```python
from build123d import *

# Parameters (mm, degrees)
F0_W     = 87.63
F0_H     = 71.12
F1_DEPTH = 25.4
F2_W     = 74.929997
F2_H     = 58.42
F3_DEPTH = 24.13
F4_W     = 16.083958
F4_H     = 6.761409
F5_DEPTH = 7.62
F6_W     = 87.63
F6_H     = 1.905
F7_DEPTH = 5.08
F9_DEPTH = 5.08


with BuildPart() as f1:
    # F0 (on Top) → F1 (new body)
    with BuildSketch(Plane.XY):
        with Locations((-1.058847, -6.879137)):
            Rectangle(F0_W, F0_H)
    extrude(amount=F1_DEPTH)

    # F2 (on face) → F3 (cut)
    with BuildSketch(Plane.XY.offset(25.4)):
        with Locations((-1.058847, -6.879137)):
            Rectangle(F2_W, F2_H)
    extrude(amount=-F3_DEPTH, mode=Mode.SUBTRACT)

    # F4 (on face) → F5 (cut)
    with BuildSketch(Plane.YZ.offset(42.756153)):
        with Locations((8.041979, 15.468483)):
            Rectangle(F4_W, F4_H)
    extrude(amount=-F5_DEPTH, mode=Mode.SUBTRACT)

    # F6 (on face) → F7 (cut)
    with BuildSketch(Plane.XY.offset(25.4)):
        with Locations((-1.058847, 25.061363)):
            Rectangle(F6_W, F6_H)
        with Locations((-1.058847, -38.819637)):
            Rectangle(F6_W, F6_H)
    extrude(amount=-F7_DEPTH, mode=Mode.SUBTRACT)

    # F8 (on face) → F9 (join)
    with BuildSketch(Plane.XY.offset(12.087778)):
        Polygon((12.600807, 0), (36.406152, 0), (36.406152, 16.083958), (36.406152, 22.332337), (12.600807, 22.332337), align=None)
    extrude(amount=-F9_DEPTH)


solid = f1.part
```
The listing builds one solid part. Answer for the finished solid, in the listing's coordinates (mm). A direction names the side the tool comes from. Round coordinates to 2 decimals unless told otherwise and drop trailing zeros. Loops run counter-clockwise (first coordinate to the right, second up) from the corner with the lowest first, then second, coordinate; pieces in that order, holes last.
Q1. Section D-D, the plane x = 27 is taken. Determine the outline of the cut face in (y, z).
Q2. Given pin 1 Ø5 at (x, y) = (16, -23) entering from +Z; pin 2 Ø6.5 at (x, y) = (19, 8) entering from +Z, each flat-ended and moving along its own axis, determine where each tip first touches the part or whether it passes through.
Q3. Find the intervals of material crossed by line 1 (Y direction, x = 18.5, z = 20.75); line 2 (X direction, y = -2.5, z = 22.25); line 3 (Z direction, x = 21, y = 12.5), in increasing order.
Q4. Section A-A, the plane z = 21.25 is taken. Determine the outline of the cut face in (x, y), then the cut area to 3 significant figures.
Q5. For a pull along X with two mould halves and no side action, classify faces 6 (the face through (-44.874, -7, 13)), 7 (the face through (-2, -6, 0)), 8 (the face through (24, 11, 12.088)) as released by +X, released by -X, zero draft, split by the parting line, or undercut.
Q6. Which of the six approach directions +Z, -Z, +X, -X, +Y, -Y give full straight-line access (tool end or side, diameter ignored) to faces 1 (the face through (-2, -39.772, 23)), 2 (the face through (12.601, 11, 10)), 3 (the face through (40, 0, 15)), 4 (the face through (-1, 23, 25.4)), 5 (the face through (-2, -6, 1.27))?
Q7. Section B-B, the plane y = 11 is taken. Determine the outline of the cut face in (x, z), then the cut area to 3 significant figures.
Q8. Section C-C, the plane z = 10.75 is taken. Determine the outline of the cut face in (x, y), then the cut area to 3 significant figures.
Completed:
1. outline: (-42.44, 0) - (28.68, 0) - (28.68, 25.4) - (26.01, 25.4) - (26.01, 20.32) - (24.11, 20.32) - (24.11, 25.4) - (22.33, 25.4) - (22.33, 12.09) - (0, 12.09) - (0, 7.01) - (22.33, 7.01) - (22.33, 1.27) - (-36.09, 1.27) - (-36.09, 25.4) - (-37.87, 25.4) - (-37.87, 20.32) - (-39.77, 20.32) - (-39.77, 25.4) - (-42.44, 25.4) - close
2. pin 1: stops at z = 1.27
2. pin 2: stops at z = 12.09
3. line 1: y = -42.44 to -39.77, -37.87 to -36.09, 22.33 to 24.11, 26.01 to 28.68
3. line 2: x = -44.87 to -38.52, 36.41 to 42.76
3. line 3: z = 0 to 1.27, 7.01 to 12.09
4. outline: (-44.87, -42.44) - (42.76, -42.44) - (42.76, -39.77) - (-44.87, -39.77) - close; (-44.87, -37.87) - (42.76, -37.87) - (42.76, 24.11) - (-44.87, 24.11) - close; (-44.87, 26.01) - (42.76, 26.01) - (42.76, 28.68) - (-44.87, 28.68) - close; hole (-38.52, -36.09) - (36.41, -36.09) - (36.41, 22.33) - (-38.52, 22.33) - close
4. area: 1,520 mm2
5. face 6: released by -X
5. face 7: zero draft
5. face 8: undercut
6. face 1: +Z, +X, -X
6. face 2: +Z
6. face 3: +X
6. face 4: +Z, +X, -X, +Y, -Y
6. face 5: none
7. outline: (-44.87, 0) - (42.76, 0) - (42.76, 12.09) - (12.6, 12.09) - (12.6, 7.01) - (36.41, 7.01) - (36.41, 1.27) - (-38.52, 1.27) - (-38.52, 25.4) - (-44.87, 25.4) - close; (36.41, 18.85) - (42.76, 18.85) - (42.76, 25.4) - (36.41, 25.4) - close
7. area: 496 mm2
8. outline: (-44.87, -42.44) - (42.76, -42.44) - (42.76, 28.68) - (-44.87, 28.68) - close; hole (-38.52, -36.09) - (36.41, -36.09) - (36.41, 0) - (12.6, 0) - (12.6, 22.33) - (-38.52, 22.33) - close
8. area: 2,390 mm2
